```python
from build123d import *

# Parameters (mm, degrees)
SKETCH1_W           = 50.8
SKETCH1_H           = 25.4
BOSS_EXTRUDE1_DEPTH = 38.1
SHELL1_T            = -3.175
SKETCH2_R           = 2.4892
CUT_EXTRUDE1_DEPTH  = 63.5


with BuildPart() as part:
    # Sketch1 → Boss-Extrude1 (new, symmetric)
    with BuildSketch(Plane.XY):
        Rectangle(SKETCH1_W, SKETCH1_H)
    extrude(amount=BOSS_EXTRUDE1_DEPTH, both=True)

    # Shell1
    shell1_openings = [part.faces().sort_by_distance(p)[0] for p in [
        (0, 0, 38.1),
        (0, 0, -38.1),
    ]]
    offset(amount=SHELL1_T, openings=shell1_openings, kind=Kind.INTERSECTION)

    # Sketch2 → Cut-Extrude1 (cut, symmetric)
    with BuildSketch(Plane(origin=(0, 0, 0), x_dir=(1, 0, 0), z_dir=(0, 1, 0))):
        with Locations(Location((-12.7, 25.4, 0), (0, 0, 270))):
            Circle(SKETCH2_R)
        with Locations(Location((12.7, 25.4, 0), (0, 0, 270))):
            Circle(SKETCH2_R)
        with Locations(Location((12.7, 12.7, 0), (0, 0, 270))):
            Circle(SKETCH2_R)
        with Locations(Location((12.7, 0, 0), (0, 0, 270))):
            Circle(SKETCH2_R)
        with Locations(Location((12.7, -12.7, 0), (0, 0, 270))):
            Circle(SKETCH2_R)
        with Locations(Location((12.7, -25.4, 0), (0, 0, 270))):
            Circle(SKETCH2_R)
        with Locations((12.7, -38.1)):
            Circle(SKETCH2_R)
        with Locations(Location((-12.7, 12.7, 0), (0, 0, 270))):
            Circle(SKETCH2_R)
        with Locations(Location((-12.7, 0, 0), (0, 0, 270))):
            Circle(SKETCH2_R)
        with Locations(Location((-12.7, -12.7, 0), (0, 0, 270))):
            Circle(SKETCH2_R)
        with Locations(Location((-12.7, -25.4, 0), (0, 0, 270))):
            Circle(SKETCH2_R)
        with Locations((-12.7, -38.1)):
            Circle(SKETCH2_R)
    extrude(amount=CUT_EXTRUDE1_DEPTH, both=True, mode=Mode.SUBTRACT)


solid = part.part
```
The model under review builds one solid part; all positions refer to its coordinate system, in mm. A direction names the side the tool comes from. Round coordinates to 2 decimals unless told otherwise and drop trailing zeros. Write each loop counter-clockwise with the first axis right and the second up, starting at its lowest first coordinate (ties: lowest second). Pieces come first, ordered by that corner, then holes. Notation, with made-up numbers: (6.25, 83.25) - (24.25, 83.25) arc R18 cw to (24.25, 98.25) - close; hole circle Ø10 at (-7.5, 67). An arc over 180 degrees is marked (long way). Use one line per item in the form item = value.
Q1. Draft analysis for pull direction Z (two halves, no side actions). For faces 3 (the flat face through (22.5, 0.2, 38.1)), 4 (the cylindrical face through (14.8, -11.09, 26.74)), 5 (the cylindrical face through (-11.952, 11.09, 27.774)), 6 (the flat face through (0, -9.525, 1)), state which applies: +Z half, -Z half, draft (parallel to the pull), parting line (faces both ways), or undercut.
Answer key:
face_3 = +Z half
face_4 = undercut
face_5 = undercut
face_6 = draft
Q2. For line 1 (X direction, y = -11.7, z = 0); line 2 (Z direction, x = 12.7, y = 11.85); line 3 (X direction, y = 8.25, z = 35.5) (3 decimals), list the stretches that pass through material, from the lowest coordinate up. Write a range as [from, to].
Answer key:
line_1 = [-25.4, -15.19], [-10.21, 10.21], [15.19, 25.4]
line_2 = [-38.1, -27.89], [-22.91, -15.19], [-10.21, -2.49], [2.49, 10.21], [15.19, 22.91], [27.89, 35.61]
line_3 = [-25.4, -22.225], [22.225, 25.4]
Q3. Consider section A-A (z = -25.4). State the section outline as (x, y) points (3 decimals), and give its area (3 significant figures).
Answer key:
outline = (-25.4, -12.7) - (-15.189, -12.7) - (-15.189, -9.525) - (-22.225, -9.525) - (-22.225, 9.525) - (-15.189, 9.525) - (-15.189, 12.7) - (-25.4, 12.7) - close; (-10.211, -12.7) - (10.211, -12.7) - (10.211, -9.525) - (-10.211, -9.525) - close; (-10.211, 9.525) - (10.211, 9.525) - (10.211, 12.7) - (-10.211, 12.7) - close; (15.189, -12.7) - (25.4, -12.7) - (25.4, 12.7) - (15.189, 12.7) - (15.189, 9.525) - (22.225, 9.525) - (22.225, -9.525) - (15.189, -9.525) - close
area = 380 mm2
Q4. Consider section B-B (x = -20.5). State the section outline as (y, z) points (3 decimals), and give its area (3 significant figures).
Answer key:
outline = (-12.7, -38.1) - (-9.525, -38.1) - (-9.525, 38.1) - (-12.7, 38.1) - close; (9.525, -38.1) - (12.7, -38.1) - (12.7, 38.1) - (9.525, 38.1) - close
area = 484 mm2
Q5. Insertion check: pin 1 Ø4 at (x, z) = (12.7, 25.4) entering from +Y. The pin has a flat end and moves straight along its axis. Give the tip position at first contact, or say it passes through.
Answer key:
pin_1 = through
Q6. Consider section D-D (x = 12.7). State how many separate pieces and enclosed holes the cut face has, and give its area (3 significant figures).
Answer key:
separate_pieces = 12
enclosed_holes = 0
area = 310 mm2
Q7. Tool access review of faces 1 (the flat face through (22.225, 0, 1)), 2 (the cylindrical face through (-10.23, 11.09, -0.32)): name each direction out of +Z, -Z, +X, -X, +Y, -Y from which nothing blocks a thin tool from reaching the whole face with its end or side.
Answer key:
face_1 = +Z, -Z
face_2 = +Y, -Y
Q8. Consider section C-C (y = -8.5). State the section outline as (x, z) points (3 decimals).
Answer key:
outline = (-25.4, -38.1) - (-22.225, -38.1) - (-22.225, 38.1) - (-25.4, 38.1) - close; (22.225, -38.1) - (25.4, -38.1) - (25.4, 38.1) - (22.225, 38.1) - close
